CAD build for the part. Positions are in the model's coordinates, mm. A direction names the side the tool comes from. Coordinates: 2 decimals unless noted, no trailing zeros. Loops run counter-clockwise (first coordinate to the right, second up) from the corner with the lowest first, then second, coordinate; pieces in that order, holes last. Notation, with made-up numbers: (35, 67.5) - (81, 67.5) arc R24 cw to (81, 91.5) - close; hole circle Ø2 at (79, -0.75). An arc over 180 degrees is marked (long way). Put each result on its own line as item: value.
```python
from build123d import *

# Parameters (mm, degrees)
SKETCH031_R        = 1.75
PAD018_DEPTH       = 10
POCKET003_DEPTH    = 2.6
PAD019_DEPTH       = 10
SKETCH034_R        = 15
PAD020_DEPTH       = 5
SKETCH035_R        = 4
POCKET004_DEPTH    = 12.7
SKETCH036_R        = 2
POCKET005_DEPTH    = 5
PAD021_DEPTH       = 5
POLARPATTERN_COUNT = 4


with BuildPart() as part:
    # Sketch031 (on Face1 of Binder005) → Pad018 (new body)
    with BuildSketch(Plane(origin=(0, 0, 0), x_dir=(1, 0, 0), z_dir=(0, 0, -1))):
        Polygon((-60.104076, 53.033009), (-53.033009, 60.104076), (53.033009, 60.104076), (60.104076, 53.033009), (60.104076, -53.033009), (53.033009, -60.104076), (-53.033009, -60.104076), (-60.104076, -53.033009), align=None)
        with Locations((-51.568542, -51.568542)):
            Circle(SKETCH031_R, mode=Mode.SUBTRACT)
        with Locations((51.568542, -51.568542)):
            Circle(SKETCH031_R, mode=Mode.SUBTRACT)
        with Locations((51.568542, 51.568542)):
            Circle(SKETCH031_R, mode=Mode.SUBTRACT)
        with Locations((-51.568542, 51.568542)):
            Circle(SKETCH031_R, mode=Mode.SUBTRACT)
        Polygon((-43.033009, 50.104076), (43.033009, 50.104076), (50.104076, 43.033009), (50.104076, -43.033009), (43.033009, -50.104076), (-43.033009, -50.104076), (-50.104076, -43.033009), (-50.104076, 43.033009), align=None, mode=Mode.SUBTRACT)
    extrude(amount=PAD018_DEPTH)

    # Sketch032 (on Face22 of Pad018) → Pocket003 (cut)
    with BuildSketch(Plane(origin=(0, 0, -10), x_dir=(1, 0, 0), z_dir=(0, 0, -1))):
        Polygon((-48.104441, -51.568542), (-49.836492, -48.568542), (-53.300593, -48.568542), (-55.032644, -51.568542), (-53.300593, -54.568542), (-49.836492, -54.568542), align=None)
        Polygon((53.300593, -48.568542), (49.836492, -48.568542), (48.104441, -51.568542), (49.836492, -54.568542), (53.300593, -54.568542), (55.032644, -51.568542), align=None)
        Polygon((53.300593, 54.568542), (49.836492, 54.568542), (48.104441, 51.568542), (49.836492, 48.568542), (53.300593, 48.568542), (55.032644, 51.568542), align=None)
        Polygon((-49.836492, 54.568542), (-53.300593, 54.568542), (-55.032644, 51.568542), (-53.300593, 48.568542), (-49.836492, 48.568542), (-48.104441, 51.568542), align=None)
    extrude(amount=-POCKET003_DEPTH, mode=Mode.SUBTRACT)

    # Sketch033 (on Face5 of Pocket003) → Pad019 (join)
    with BuildSketch(Plane(origin=(0, 0, -10), x_dir=(1, 0, 0), z_dir=(0, 0, -1))):
        with BuildLine():
            Line((-43.033009, -50.104076), (-6.464466, -13.535534))
            ThreePointArc((-6.464466, -13.535534), (0, -15), (6.464466, -13.535534))
            Line((43.033009, -50.104076), (6.464466, -13.535534))
            Line((50.104076, -43.033009), (43.033009, -50.104076))
            Line((50.104076, -43.033009), (13.535534, -6.464466))
            ThreePointArc((13.535534, -6.464466), (15, 0), (13.535534, 6.464466))
            Line((50.104076, 43.033009), (13.535534, 6.464466))
            Line((43.033009, 50.104076), (50.104076, 43.033009))
            Line((43.033009, 50.104076), (6.464466, 13.535534))
            ThreePointArc((6.464466, 13.535534), (0, 15), (-6.464466, 13.535534))
            Line((-43.033009, 50.104076), (-6.464466, 13.535534))
            Line((-50.104076, 43.033009), (-43.033009, 50.104076))
            Line((-50.104076, 43.033009), (-13.535534, 6.464466))
            ThreePointArc((-13.535534, 6.464466), (-15, 0), (-13.535534, -6.464466))
            Line((-50.104076, -43.033009), (-13.535534, -6.464466))
            Line((-43.033009, -50.104076), (-50.104076, -43.033009))
        make_face()
    extrude(amount=-PAD019_DEPTH)

    # Sketch034 (on Face32 of Pad019) → Pad020 (join)
    with BuildSketch(Plane(origin=(0, 0, -10), x_dir=(1, 0, 0), z_dir=(0, 0, -1))):
        Circle(SKETCH034_R)
    extrude(amount=PAD020_DEPTH)

    # Sketch035 (on Face65 of Pad020) → Pocket004 (cut)
    with BuildSketch(Plane(origin=(0, 0, -15), x_dir=(1, 0, 0), z_dir=(0, 0, -1))):
        Circle(SKETCH035_R)
    extrude(amount=-POCKET004_DEPTH, mode=Mode.SUBTRACT)

    # Sketch036 (on Face65 of Pocket004) → Pocket005 (cut)
    with BuildSketch(Plane(origin=(0, 0, -15), x_dir=(1, 0, 0), z_dir=(0, 0, -1))):
        with Locations((13, 0)):
            Circle(SKETCH036_R)
    extrude(amount=-POCKET005_DEPTH, mode=Mode.SUBTRACT)

    # Sketch039 (on DatumPlane) → Pad021 (join, symmetric)
    with BuildSketch(Plane(origin=(53.235209, -53.235209, -8.333333), x_dir=(0.707107, -0.707107, 0), z_dir=(-0.707107, -0.707107, 0))):
        Polygon((-9.42809, -1.666667), (-63.285955, -1.666667), (-63.285955, -6.666667), (-60.285955, -6.666667), align=None)
    pad021 = extrude(amount=PAD021_DEPTH, both=True)

    # PolarPattern: Pad021 ×4 about axis
    polarpattern_axis = Axis((0, 0, 0), (0, 0, 1))
    for i in range(1, POLARPATTERN_COUNT):
        add(pad021.rotate(polarpattern_axis, i * 360 / POLARPATTERN_COUNT))


solid = part.part
```
Q1. Slice it at B-B, the plane y = 46. Give the cut face in (x, z).
Determined:
outline: (-60.1, -10) - (-47.14, -10) - (-38.93, -10.57) - (-38.93, 0) - (-60.1, 0) - close; (38.93, -10.57) - (47.14, -10) - (60.1, -10) - (60.1, 0) - (38.93, 0) - close
Q2. Wall check: L1, parallel to Y at x = 50.5, z = -9; L2, parallel to X at y = 0, z = -9.5; L3, parallel to X at y = 3, z = -8.5. Give the ranges that are in metal, low to high. Write a range as from..to.
Determined:
L1: -60.1..-54.57, -48.57..48.57, 54.57..60.1
L2: -60.1..-50.1, -15..-4, 4..15, 50.1..60.1
L3: -60.1..-50.1, -14.7..-2.65, 2.65..14.7, 50.1..60.1
Q3. Pin check, flat tips, straight feed: pin 1 Ø6.5 at (x, y) = (0, 0) entering from -Z; pin 2 Ø2 at (x, y) = (51.57, 51.57) entering from +Z; pin 3 Ø5.5 at (x, y) = (51.57, -51.57) entering from -Z; pin 4 Ø3 at (x, y) = (13, 0) entering from -Z. Stop position of each tip, or through.
Determined:
pin 1: z = -2.3
pin 2: through
pin 3: z = -7.4
pin 4: z = -10
Q4. Tool access for faces 4 (the flat face through (1, 50.104, -5)), 5 (the flat face through (56.618, 56.519, -4.93)), 6 (the flat face through (-54.154, 50.048, -8.718)): list every direction of +Z, -Z, +X, -X, +Y, -Y with a clear straight run to the whole face (end or side of a thin tool).
Determined:
face 4: +Z, -Z
face 5: +Z, -Z, +X, +Y
face 6: -Z
Q5. Slice it at A-A, the plane x = 0. Give the cut face in (y, z), then the cut area to 3 significant figures.
Determined:
outline: (-60.1, -10) - (-50.1, -10) - (-50.1, 0) - (-60.1, 0) - close; (-15, -15) - (-4, -15) - (-4, -2.3) - (4, -2.3) - (4, -15) - (15, -15) - (15, 0) - (-15, 0) - close; (50.1, -10) - (60.1, -10) - (60.1, 0) - (50.1, 0) - close
area: 548 mm2
Q6. Slice it at D-D, the plane x = 32.5. Give the cut face in (y, z).
Determined:
outline: (-60.1, -10) - (-50.1, -10) - (-50.1, 0) - (-60.1, 0) - close; (-39.57, -11.46) - (-25.43, -12.45) - (-25.43, 0) - (-39.57, 0) - close; (25.43, -12.45) - (39.57, -11.46) - (39.57, 0) - (25.43, 0) - close; (50.1, -10) - (60.1, -10) - (60.1, 0) - (50.1, 0) - close
Q7. Slice it at C-C, the plane z = -4.5. State how many separate pieces and enclosed holes the cut face has, then the cut area to 3 significant figures.
Determined:
separate pieces: 1
enclosed holes: 9
area: 7,070 mm2
Q8. Mould opens along Y. For faces 1 (the flat face through (60.104, -1, -5)), 2 (the flat face through (56.519, -56.618, -4.93)), 3 (the flat face through (52, 48.569, -9)) say: +Y half, -Y half, draft (parallel to the pull), parting line (faces both ways), or undercut.
Determined:
face 1: draft
face 2: -Y half
face 3: undercut
